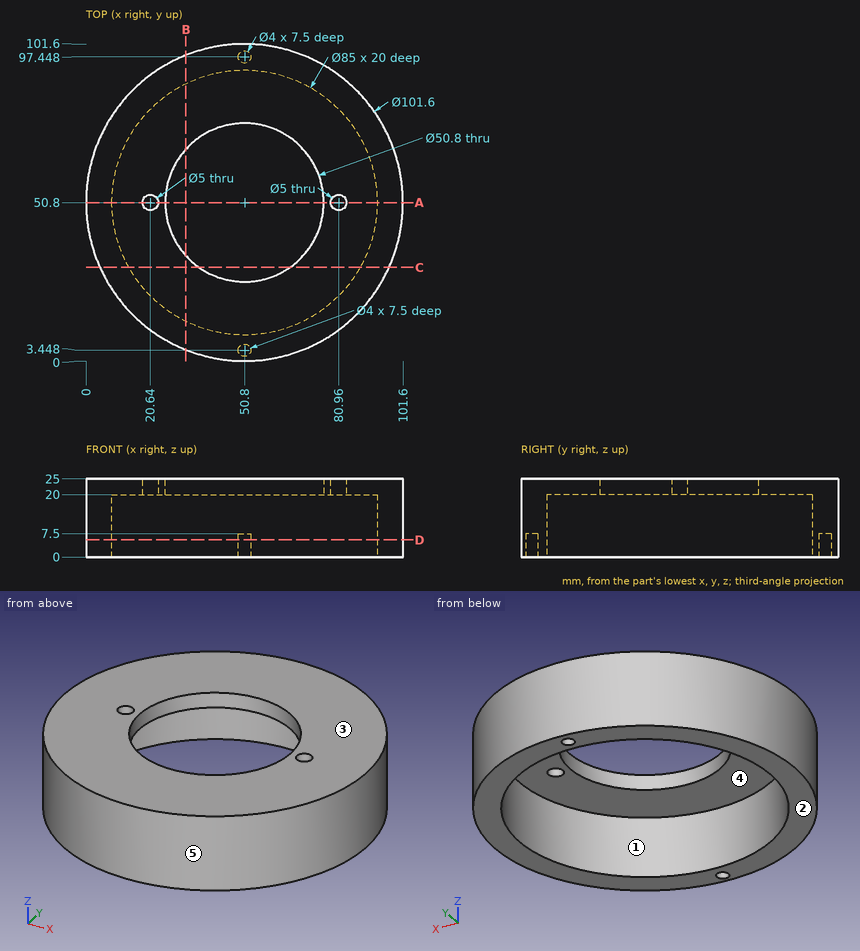
Input: dimensioned drawing with shaded views. Units: mm. Origin: part minimum x, y, z. A direction names the side the tool comes from. Coordinates: 2 decimals unless noted, no trailing zeros. Write each loop counter-clockwise with the first axis right and the second up, starting at its lowest first coordinate (ties: lowest second). Pieces come first, ordered by that corner, then holes. Notation, with made-up numbers: (89.5, 24) -> (110.5, 24) arc R30 cw to (110.5, 52) -> close; hole circle Ø11 at (-18, -9). An arc over 180 degrees is marked (long way). Return JSON: item names as keys, results as strings. Group by question number.
1) Ray query, line 1 along Y through (x, z) = (50.8, 5.75); line 2 along Y through (x, z) = (50.8, 21.7); line 3 along Z through (x, y) = (38, 85.5). Return the intervals inside material, ascending.
2) Section query C-C, the plane y = 30. Return loops of the section in (x, z), plus the area to 3 significant figures.
3) Contact query for flat-ended pins moving along their axis: P1, Ø4, axis at y = 77.5, z = 18.5, coming from the -X side; P2, Ø12, axis at y = 22.5, z = 14.5, coming from the +X side; P3, Ø12, axis at x = 23, z = 6, coming from the +Y side (1 decimal). Output: stop coordinate, or through.
4) Section query D-D, the plane z = 5.5. Return loops of the section in (x, y), plus the area to 3 significant figures.
5) Section query A-A, the plane y = 50.8. Return loops of the section in (x, z), plus the area to 3 significant figures.
6) Mould query, pull axis X, two halves, no side actions, for the marked faces 3, 4 and 5. Classes: +X half, -X half, draft (parallel to the pull), parting line (faces both ways), or undercut.
7) Set-up query: the marked faces 1 and 2. Return all of +Z, -Z, +X, -X, +Y, -Y with unobstructed straight access to the full face (end or side cutting, diameter ignored); none if empty.
8) Section query B-B, the plane x = 32. Return loops of the section in (y, z) (1 decimal), plus the area to 3 significant figures.
From the geometry:
{
 "1": {"line 1": "0 to 1.45, 5.45 to 8.3, 93.3 to 95.45, 99.45 to 101.6", "line 2": "0 to 25.4, 76.2 to 101.6", "line 3": "20 to 25"},
 "2": {"outline": "(4.45, 0) -> (13.74, 0) -> (13.74, 20) -> (36.22, 20) -> (36.22, 25) -> (4.45, 25) -> close; (65.38, 20) -> (87.86, 20) -> (87.86, 0) -> (97.15, 0) -> (97.15, 25) -> (65.38, 25) -> close", "area": "689 mm²"},
 "3": {"P1": "x = 6.41", "P2": "x = 96.44", "P3": "y = 96.7"},
 "4": {"outline": "circle Ø101.6 at (50.8, 50.8); hole circle Ø85 at (50.8, 50.8); hole circle Ø4 at (50.8, 3.45); hole circle Ø4 at (50.8, 97.45)", "area": "2,410 mm²"},
 "5": {"outline": "(0, 0) -> (8.3, 0) -> (8.3, 20) -> (18.14, 20) -> (18.14, 25) -> (0, 25) -> close; (23.14, 20) -> (25.4, 20) -> (25.4, 25) -> (23.14, 25) -> close; (76.2, 20) -> (78.46, 20) -> (78.46, 25) -> (76.2, 25) -> close; (83.46, 20) -> (93.3, 20) -> (93.3, 0) -> (101.6, 0) -> (101.6, 25) -> (83.46, 25) -> close", "area": "536 mm²"},
 "6": {"face 3": "draft", "face 4": "undercut", "face 5": "parting line"},
 "7": {"face 1": "-Z", "face 2": "-Z, +X, -X, +Y, -Y"},
 "8": {"outline": "(3.6, 0) -> (12.7, 0) -> (12.7, 20) -> (33.7, 20) -> (33.7, 25) -> (3.6, 25) -> close; (67.9, 20) -> (88.9, 20) -> (88.9, 0) -> (98, 0) -> (98, 25) -> (67.9, 25) -> close", "area": "664 mm²"}
}
